Read the model definition and answer for the solid it produces. Units are mm, in the model's axes. Face numbers are marked on the shaded views. A direction names the side the tool comes from. Give positions to 0.01 mm unless a question says otherwise; leave off trailing zeros. Loops run counter-clockwise (first coordinate to the right, second up) from the corner with the lowest first, then second, coordinate; pieces in that order, holes last. Notation, with made-up numbers: (54.5, -9) - (94.5, -9) arc R20 ccw to (94.5, 13) - close; hole circle Ø6 at (48.5, 81). An arc over 180 degrees is marked (long way). Use a Markdown table: item, result. Add a question column.
Item 1: A cutting plane is placed at C-C (z = -7.5). Determine the outline of the cut face in (x, y), plus the area to 3 significant figures.
Item 2: Each of these flat-tipped pins is pushed along its axis until it touches: P1, Ø4, axis at x = 6, z = 9, coming from the +Y side; P2, Ø1, axis at x = 9.5, z = 6, coming from the +Y side; P3, Ø2, axis at x = 9, z = 0.5, coming from the -Y side. Where does it stop, or does it pass through?
Item 3: Which of the six approach directions +Z, -Z, +X, -X, +Y, -Y give full straight-line access (tool end or side, diameter ignored) to the marked faces 1, 2 and 3?
Item 4: A cutting plane is placed at B-B (x = 1.75). Determine the outline of the cut face in (y, z).
Item 5: A cutting plane is placed at D-D (x = 3.5). Determine the outline of the cut face in (y, z).
Item 6: Consider probe 1 along Z at (x, y) = (7, 7.25); probe 2 along X at (y, z) = (-1.5, -7); probe 3 along Y at (x, z) = (3, -8.5). Determine where each line is inside the solid, lowest interval first. Write a range as [from, to].
Item 7: A cutting plane is placed at A-A (y = 0). Determine the outline of the cut face in (x, z), plus the area to 3 significant figures.
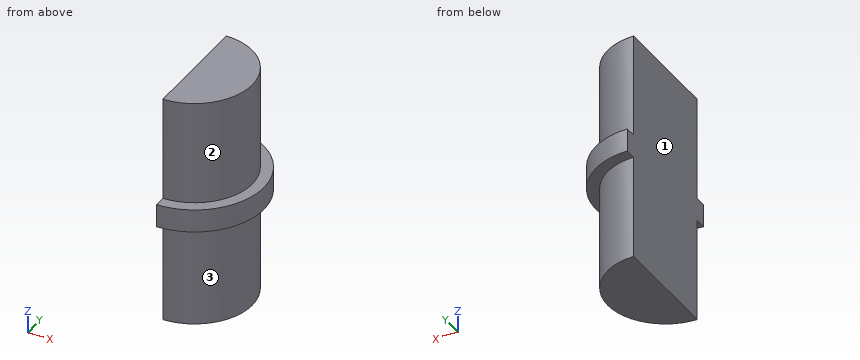
from build123d import *

# Parameters (mm, degrees)
F0_W     = 2
F0_H     = 2
F1_ANGLE = 180


with BuildPart() as f1:
    # F0 (on Front) → F1 (revolve, symmetric)
    with BuildSketch(Plane.XZ) as f1_sk:
        Polygon((0, 20), (0, 0), (0, -20), (10, -20), (10, -2), (10, 0), (10, 2), (10, 20), align=None)
        with Locations((11, -1)):
            Rectangle(F0_W, F0_H)
        with Locations((11, 1)):
            Rectangle(F0_W, F0_H)
    revolve(axis=Axis((0, 0, 10), (0, 0, 1)), revolution_arc=F1_ANGLE / 2)
    revolve(f1_sk.sketch, axis=Axis((0, 0, 10), (0, 0, -1)), revolution_arc=F1_ANGLE / 2)


solid = f1.part
Geometry says:
| question | item | result |
|---|---|---|
| 1 | outline | (0, -10) arc R10 ccw to (0, 10) - close |
| 1 | area | 157 mm² |
| 2 | P1 | y = 9.17 |
| 2 | P2 | y = 4.36 |
| 2 | P3 | y = -8.94 |
| 3 | face 1 | +Z, -Z, -X, +Y, -Y |
| 3 | face 2 | +Z, +X |
| 3 | face 3 | -Z, +X |
| 4 | outline | (-11.87, -2) - (-9.85, -2) - (-9.85, -20) - (9.85, -20) - (9.85, -2) - (11.87, -2) - (11.87, 2) - (9.85, 2) - (9.85, 20) - (-9.85, 20) - (-9.85, 2) - (-11.87, 2) - close |
| 5 | outline | (-11.48, -2) - (-9.37, -2) - (-9.37, -20) - (9.37, -20) - (9.37, -2) - (11.48, -2) - (11.48, 2) - (9.37, 2) - (9.37, 20) - (-9.37, 20) - (-9.37, 2) - (-11.48, 2) - close |
| 6 | probe 1 | [-2, 2] |
| 6 | probe 2 | [0, 9.89] |
| 6 | probe 3 | [-9.54, 9.54] |
| 7 | outline | (0, -20) - (10, -20) - (10, -2) - (12, -2) - (12, 2) - (10, 2) - (10, 20) - (0, 20) - close |
| 7 | area | 408 mm² |
